```python
from build123d import *

# Parameters (mm, degrees)
SKETCH_1_R          = 1.6
SKETCH_1_R_2        = 7.5
EXTRUDE_1_DEPTH     = 6.5
EXTRUDE_2_DEPTH     = 50
SKETCH_3_R          = 2.5
CUT_EXTRUDE_1_DEPTH = 10
CUT_EXTRUDE_2_REACH = 108.546
SKETCH_5_R          = 2.5
CUT_EXTRUDE_3_REACH = 108.469
SKETCH_6_R          = 2.5


with BuildPart() as part:
    # 草图1 → 凸台-拉伸1 (new body)
    with BuildSketch(Plane.XY):
        with BuildLine():
            Line((-36.800051208, 35), (38.850303739, 35))
            ThreePointArc((38.850303739, 35), (51.648918374, 29.698640239), (56.950278135, 16.900025604))
            Line((56.950278135, 16.900025604), (56.950278135, -16.900025604))
            ThreePointArc((56.950278135, -16.900025604), (50.945911029, -30.48186799), (36.800051208, -35))
            Line((36.800051208, -35), (-36.800051208, -35))
            ThreePointArc((-36.800051208, -35), (-49.598665842, -29.698640239), (-54.900025604, -16.900025604))
            Line((-54.900025604, -16.900025604), (-54.900025604, 16.900025604))
            ThreePointArc((-54.900025604, 16.900025604), (-49.598665842, 29.698640239), (-36.800051208, 35))
        make_face()
        with Locations(Location((-50.400025604, 16.900025604, 0), (0, 0, 180))):
            Circle(SKETCH_1_R, mode=Mode.SUBTRACT)
        with Locations(Location((-40.000025604, 10.900025604, 0), (0, 0, 180))):
            Circle(SKETCH_1_R_2, mode=Mode.SUBTRACT)
        with Locations(Location((52.450278135, 16.900025604, 0), (0, 0, 180))):
            Circle(SKETCH_1_R, mode=Mode.SUBTRACT)
        with Locations(Location((42.050278135, 10.900025604, 0), (0, 0, 180))):
            Circle(SKETCH_1_R_2, mode=Mode.SUBTRACT)
        with Locations(Location((52.450278135, -16.900025604, 0), (0, 0, 180))):
            Circle(SKETCH_1_R, mode=Mode.SUBTRACT)
        with Locations(Location((-50.400025604, -16.900025604, 0), (0, 0, 180))):
            Circle(SKETCH_1_R, mode=Mode.SUBTRACT)
        with BuildLine():
            Line((-15.5, 22.5), (15.5, 22.5))
            ThreePointArc((15.5, 22.5), (20.449747468, 20.449747468), (22.5, 15.5))
            Line((22.5, 15.5), (22.5, -15.5))
            ThreePointArc((22.5, -15.5), (20.449747468, -20.449747468), (15.5, -22.5))
            Line((15.5, -22.5), (-15.5, -22.5))
            ThreePointArc((-15.5, -22.5), (-20.449747468, -20.449747468), (-22.5, -15.5))
            Line((-22.5, -15.5), (-22.5, 15.5))
            ThreePointArc((-22.5, 15.5), (-20.449747468, 20.449747468), (-15.5, 22.5))
        make_face(mode=Mode.SUBTRACT)
    extrude(amount=EXTRUDE_1_DEPTH)

    # 草图2 → 凸台-拉伸2 (add)
    with BuildSketch(Plane.XY.offset(6.5)):
        with BuildLine():
            Line((8.843450288, -22.5), (-8.843450288, -22.5))
            ThreePointArc((-8.843450288, -22.5), (-11.48607102, -23.92742014), (-12.539948379, -26.739948379))
            Line((-12.539948379, -26.739948379), (-12.539948379, -35))
            Line((-12.539948379, -35), (12.539948379, -35))
            Line((12.539948379, -35), (12.539948379, -26.739948379))
            ThreePointArc((12.539948379, -26.739948379), (11.48607102, -23.92742014), (8.843450288, -22.5))
        make_face()
        with BuildLine():
            Line((-20.8, 22.5), (20.8, 22.5))
            ThreePointArc((20.8, 22.5), (23.769848481, 23.730151519), (25, 26.7))
            Line((25, 26.7), (25, 35))
            Line((25, 35), (-25, 35))
            Line((-25, 35), (-25, 26.7))
            ThreePointArc((-25, 26.7), (-23.769848481, 23.730151519), (-20.8, 22.5))
        make_face()
    extrude(amount=EXTRUDE_2_DEPTH)

    # 草图3 → 切除-拉伸1 (cut)
    with BuildSketch(Plane.XY.offset(56.5)):
        with Locations((-12, 28.75)):
            Circle(SKETCH_3_R)
        with Locations((12, 28.75)):
            Circle(SKETCH_3_R)
        with Locations((-6, -28.75)):
            Circle(SKETCH_3_R)
        with Locations((6, -28.75)):
            Circle(SKETCH_3_R)
    extrude(amount=-CUT_EXTRUDE_1_DEPTH, mode=Mode.SUBTRACT)

    # 草图5 → 切除-拉伸2 (cut, up to next)
    with BuildSketch(Plane(origin=(0, 35, 0), x_dir=(1, 0, 0), z_dir=(0, 1, 0)), mode=Mode.PRIVATE) as cut_extrude_2_sk1:
        with Locations(Location((12, -20, 0), (0, 0, 180))):
            Circle(SKETCH_5_R)
    cut_extrude_2_tool1 = extrude(cut_extrude_2_sk1.sketch, amount=-CUT_EXTRUDE_2_REACH, mode=Mode.PRIVATE) & part.part
    # 草图5 → 切除-拉伸2 (cut, up to next)
    with BuildSketch(Plane(origin=(0, 35, 0), x_dir=(1, 0, 0), z_dir=(0, 1, 0)), mode=Mode.PRIVATE) as cut_extrude_2_sk2:
        with Locations((-12, -20)):
            Circle(SKETCH_5_R)
    cut_extrude_2_tool2 = extrude(cut_extrude_2_sk2.sketch, amount=-CUT_EXTRUDE_2_REACH, mode=Mode.PRIVATE) & part.part
    # 草图5 → 切除-拉伸2 (cut, up to next)
    with BuildSketch(Plane(origin=(0, 35, 0), x_dir=(1, 0, 0), z_dir=(0, 1, 0)), mode=Mode.PRIVATE) as cut_extrude_2_sk3:
        with Locations(Location((12, -36.5, 0), (0, 0, 180))):
            Circle(SKETCH_5_R)
    cut_extrude_2_tool3 = extrude(cut_extrude_2_sk3.sketch, amount=-CUT_EXTRUDE_2_REACH, mode=Mode.PRIVATE) & part.part
    # 草图5 → 切除-拉伸2 (cut, up to next)
    with BuildSketch(Plane(origin=(0, 35, 0), x_dir=(1, 0, 0), z_dir=(0, 1, 0)), mode=Mode.PRIVATE) as cut_extrude_2_sk4:
        with Locations((-12, -36.5)):
            Circle(SKETCH_5_R)
    cut_extrude_2_tool4 = extrude(cut_extrude_2_sk4.sketch, amount=-CUT_EXTRUDE_2_REACH, mode=Mode.PRIVATE) & part.part
    add(cut_extrude_2_tool1.solids().sort_by_distance((12, 35, 20))[0], mode=Mode.SUBTRACT)
    add(cut_extrude_2_tool2.solids().sort_by_distance((-12, 35, 20))[0], mode=Mode.SUBTRACT)
    add(cut_extrude_2_tool3.solids().sort_by_distance((12, 35, 36.5))[0], mode=Mode.SUBTRACT)
    add(cut_extrude_2_tool4.solids().sort_by_distance((-12, 35, 36.5))[0], mode=Mode.SUBTRACT)

    # 草图6 → 切除-拉伸3 (cut, up to next)
    with BuildSketch(Plane.XZ.offset(35), mode=Mode.PRIVATE) as cut_extrude_3_sk1:
        with Locations((-6, 20)):
            Circle(SKETCH_6_R)
    cut_extrude_3_tool1 = extrude(cut_extrude_3_sk1.sketch, amount=-CUT_EXTRUDE_3_REACH, mode=Mode.PRIVATE) & part.part
    # 草图6 → 切除-拉伸3 (cut, up to next)
    with BuildSketch(Plane.XZ.offset(35), mode=Mode.PRIVATE) as cut_extrude_3_sk2:
        with Locations((6, 20)):
            Circle(SKETCH_6_R)
    cut_extrude_3_tool2 = extrude(cut_extrude_3_sk2.sketch, amount=-CUT_EXTRUDE_3_REACH, mode=Mode.PRIVATE) & part.part
    # 草图6 → 切除-拉伸3 (cut, up to next)
    with BuildSketch(Plane.XZ.offset(35), mode=Mode.PRIVATE) as cut_extrude_3_sk3:
        with Locations((-6, 36.5)):
            Circle(SKETCH_6_R)
    cut_extrude_3_tool3 = extrude(cut_extrude_3_sk3.sketch, amount=-CUT_EXTRUDE_3_REACH, mode=Mode.PRIVATE) & part.part
    # 草图6 → 切除-拉伸3 (cut, up to next)
    with BuildSketch(Plane.XZ.offset(35), mode=Mode.PRIVATE) as cut_extrude_3_sk4:
        with Locations((6, 36.5)):
            Circle(SKETCH_6_R)
    cut_extrude_3_tool4 = extrude(cut_extrude_3_sk4.sketch, amount=-CUT_EXTRUDE_3_REACH, mode=Mode.PRIVATE) & part.part
    add(cut_extrude_3_tool1.solids().sort_by_distance((-6, -35, 20))[0], mode=Mode.SUBTRACT)
    add(cut_extrude_3_tool2.solids().sort_by_distance((6, -35, 20))[0], mode=Mode.SUBTRACT)
    add(cut_extrude_3_tool3.solids().sort_by_distance((-6, -35, 36.5))[0], mode=Mode.SUBTRACT)
    add(cut_extrude_3_tool4.solids().sort_by_distance((6, -35, 36.5))[0], mode=Mode.SUBTRACT)


solid = part.part
```
Could you check a few things on this model? Use its own coordinates, in mm. A direction names the side the tool comes from. Round coordinates to 2 decimals unless told otherwise and drop trailing zeros. Loops run counter-clockwise (first coordinate to the right, second up) from the corner with the lowest first, then second, coordinate; pieces in that order, holes last. Notation, with made-up numbers: M 55,-22.5 L 96,-22.5 A22 cw 96,11.5 Z; hole C 76.5,79.5 d3. An arc over 180 degrees is marked long. Write item = value, one per line.
1. I want a section at D-D, the plane y = 0.5. Write out the boundary of the cut face in (x, z), and give its area (3 significant figures).
Results below:
outline = M -54.9,0 L -22.5,0 L -22.5,6.5 L -54.9,6.5 Z; M 22.5,0 L 56.95,0 L 56.95,6.5 L 22.5,6.5 Z
area = 435 mm²
2. I want a section at C-C, the plane z = 43. Write out the boundary of the cut face in (x, y), and give its area (3 significant figures).
Results below:
outline = M -25,26.7 A4.2 ccw -20.8,22.5 L 20.8,22.5 A4.2 ccw 25,26.7 L 25,35 L -25,35 Z; M -12.54,-35 L 12.54,-35 L 12.54,-26.74 A4.28 ccw 8.84,-22.5 L -8.84,-22.5 A4.28 ccw -12.54,-26.74 Z
area = 923 mm²
3. I want a section at A-A, the plane x = -2. Write out the boundary of the cut face in (y, z), and give its area (3 significant figures).
Results below:
outline = M -35,0 L -22.5,0 L -22.5,56.5 L -35,56.5 Z; M 22.5,0 L 35,0 L 35,56.5 L 22.5,56.5 Z
area = 1,410 mm²
4. I need wall thicknesses on probe 1 along Y at (x, z) = (-3.5, 42.5); probe 2 along Z at (x, y) = (6, -26); probe 3 along Y at (x, z) = (-10, 48.5). Which ranges of each line are inside material? Lowest first, please.
Results below:
probe_1 = -35 to -22.5, 22.5 to 35
probe_2 = 0 to 17.5, 22.5 to 34, 39 to 56.5
probe_3 = -35 to -22.83, 22.5 to 27.25, 30.25 to 35
5. I want a section at B-B, the plane z = 36.5. Write out the boundary of the cut face in (x, y).
Results below:
outline = M -25,26.7 A4.2 ccw -20.8,22.5 L -14.5,22.5 L -14.5,35 L -25,35 Z; M -12.54,-35 L -8.5,-35 L -8.5,-22.5 L -8.84,-22.5 A4.28 ccw -12.54,-26.74 Z; M -9.5,22.5 L 9.5,22.5 L 9.5,35 L -9.5,35 Z; M -3.5,-35 L 3.5,-35 L 3.5,-22.5 L -3.5,-22.5 Z; M 8.5,-35 L 12.54,-35 L 12.54,-26.74 A4.28 ccw 8.84,-22.5 L 8.5,-22.5 Z; M 14.5,22.5 L 20.8,22.5 A4.2 ccw 25,26.7 L 25,35 L 14.5,35 Z
6. Which directions (+Z, -Z, +X, -X, +Y, -Y) give clear straight access to the entire face, cutting with the end or side of a thin tool? Please do faces 5 (the face through (-11.46, -23.9, 31.15)), 6 (the face through (12.54, -31, 31)), 7 (the face through (20.5, -20.4, 3.2)), 8 (the face through (12.54, 28.84, 34.06)).
Results below:
face_5 = +Z, -X
face_6 = +Z, +X, -Y
face_7 = +Z, -Z
face_8 = +Y
7. Will these pins go through, and if not, where does the flat tip stop? P1, Ø4.5, axis at x = -12, z = 36.5, coming from the -Y side; P2, Ø3.5, axis at x = 52.45, y = -16.9, coming from the -Z side; P3, Ø3, axis at y = 27, z = 34, coming from the -X side; P4, Ø9, axis at y = 30.5, z = 41.5, coming from the +X side.
Results below:
P1 = -35
P2 = 0
P3 = -25
P4 = 25
8. Thinking about a two-plate mould opening in X: for faces 1 (the face through (0, 29, 56.5)), 2 (the face through (20.4, 20.5, 3.2)), 3 (the face through (23.74, 23.7, 31.15)), 4 (the face through (-20.5, 20.4, 3.2)), which applies, +X half, -X half, draft (parallel to the pull), parting line (faces both ways), or undercut?
Results below:
face_1 = draft
face_2 = undercut
face_3 = +X half
face_4 = undercut
